from build123d import *

# Parameters (mm, degrees)
ESQUISSE1_W             = 20
ESQUISSE1_H             = 13.5
BOSS_EXTRU_1_DEPTH      = 2
ESQUISSE1_2_W           = 22
ESQUISSE1_2_H           = 15.5
ESQUISSE1_2_W_2         = 20
ESQUISSE1_2_H_2         = 13.5
EXTRU_MINCE1_DEPTH      = 10
ESQUISSE2_W             = 4.5
ESQUISSE2_H             = 9
ENL_V_MAT_EXTRU_1_DEPTH = 10
CONG_1_R                = 1
CONG_2_R                = 1


with BuildPart() as part:
    # Esquisse1 → Boss.-Extru.1 (new body)
    with BuildSketch(Plane.XY):
        with Locations((10, 6.75)):
            Rectangle(ESQUISSE1_W, ESQUISSE1_H)
    extrude(amount=BOSS_EXTRU_1_DEPTH)

    # Esquisse1<2> → Extru.-Mince1 (add)
    with BuildSketch(Plane.XY):
        with Locations((10, 6.75)):
            Rectangle(ESQUISSE1_2_W, ESQUISSE1_2_H)
        with Locations((10, 6.75)):
            Rectangle(ESQUISSE1_2_W_2, ESQUISSE1_2_H_2, mode=Mode.SUBTRACT)
    extrude(amount=EXTRU_MINCE1_DEPTH)

    # Esquisse2 → Enlèv. mat.-Extru.1 (cut)
    with BuildSketch(Plane.XY.offset(2)):
        with Locations((3.25, 7.25)):
            Rectangle(ESQUISSE2_W, ESQUISSE2_H)
    extrude(amount=-ENL_V_MAT_EXTRU_1_DEPTH, mode=Mode.SUBTRACT)

    # Congé1
    cong_1_edges = [part.edges().sort_by_distance(p)[0] for p in [
        (0, 0, 6),
        (20, 0, 6),
        (20, 13.5, 6),
        (0, 13.5, 6),
        (-1, 14.5, 5),
        (-1, -1, 5),
        (21, -1, 5),
        (21, 14.5, 5),
    ]]
    fillet(cong_1_edges, radius=CONG_1_R)

    # Congé2
    cong_2_edges = [part.edges().sort_by_distance(p)[0] for p in [
        (10, -1, 0),
        (-1, 6.75, 0),
        (10, 14.5, 0),
        (21, 6.75, 0),
        (20.707106781, 14.207106781, 0),
        (20.707106781, -0.707106781, 0),
        (-0.707106781, 14.207106781, 0),
        (-0.7071067811865479, -0.7071067811865458, 0),
    ]]
    fillet(cong_2_edges, radius=CONG_2_R)


solid = part.part
Could you check a few things on this model? Use its own coordinates, in mm. A direction names the side the tool comes from. Round coordinates to 2 decimals unless told otherwise and drop trailing zeros. Order: outer loops, then holes, each group sorted by start corner. A loop starts at its lowest first (then second) coordinate and runs counter-clockwise, first axis right, second up.
(1) Imagine slicing it at C-C (x = 2.75). Write out the boundary of the cut face in (y, z).
Response values:
outline: (-1, 1) arc R1 ccw to (0, 0) - (2.75, 0) - (2.75, 2) - (0, 2) - (0, 10) - (-1, 10) - close; (11.75, 0) - (13.5, 0) arc R1 ccw to (14.5, 1) - (14.5, 10) - (13.5, 10) - (13.5, 2) - (11.75, 2) - close
(2) Imagine slicing it at D-D (x = 6.5). Write out the boundary of the cut face in (y, z), plus the area to 3 significant figures.
Response values:
outline: (-1, 1) arc R1 ccw to (0, 0) - (13.5, 0) arc R1 ccw to (14.5, 1) - (14.5, 10) - (13.5, 10) - (13.5, 2) - (0, 2) - (0, 10) - (-1, 10) - close
area: 46.6 mm2
(3) If we mould it in two halves opening along Y, with no side actions, what happens to faces 4 (the flat face through (1, 7, 1)), 5 (the cylindrical face through (-0.699, 6.656, 0.285)), 6 (the cylindrical face through (10.14, -0.699, 0.285))? For each: released by +Y, released by -Y, zero draft, split by the parting line, or undercut.
Response values:
face 4: undercut
face 5: zero draft
face 6: released by -Y
(4) Please list where these lines run through material, in increasing order: line 1 along X through (y, z) = (10.75, 8); line 2 along Y through (x, z) = (6, 6); line 3 along Z through (x, y) = (11.75, 8.25).
Response values:
line 1: x = -1 to 0, 20 to 21
line 2: y = -1 to 0, 13.5 to 14.5
line 3: z = 0 to 2
(5) I'm going to push a flat-ended pin straight in: pin 1 (7 mm diameter, centred on x = 8.5, y = 8, fed in from +Z). Where does the tip first touch, or does it pass through?
Response values:
pin 1: stops at z = 2
(6) Imagine slicing it at A-A (y = 7). Write out the boundary of the cut face in (x, z).
Response values:
outline: (-1, 1) arc R1 ccw to (0, 0) - (1, 0) - (1, 2) - (0, 2) - (0, 10) - (-1, 10) - close; (5.5, 0) - (20, 0) arc R1 ccw to (21, 1) - (21, 10) - (20, 10) - (20, 2) - (5.5, 2) - close
(7) Which directions (+Z, -Z, +X, -X, +Y, -Y) give clear straight access to the entire face, cutting with the end or side of a thin tool? Please do faces 1 (the flat face through (10, 0, 6)), 2 (the flat face through (10, 14.5, 5)), 3 (the flat face through (3, 11.75, 1)).
Response values:
face 1: +Z
face 2: +Z, -Z, +X, -X, +Y
face 3: +Z, -Z
(8) Imagine slicing it at B-B (z = 6.75). Write out the boundary of the cut face in (x, y), plus the area to 3 significant figures.
Response values:
outline: (-1, 0) arc R1 ccw to (0, -1) - (20, -1) arc R1 ccw to (21, 0) - (21, 13.5) arc R1 ccw to (20, 14.5) - (0, 14.5) arc R1 ccw to (-1, 13.5) - close; hole (0, 1) arc R1 ccw to (1, 0) - (19, 0) arc R1 ccw to (20, 1) - (20, 12.5) arc R1 ccw to (19, 13.5) - (1, 13.5) arc R1 ccw to (0, 12.5) - close
area: 71.0 mm2
